Autodesk Inventor part; units mm, degrees
ref_plane "YZ Plane" through (0, 0, 0) normal (1, 0, 0) x (0, 1, 0)
ref_plane "XY Plane" through (0, 0, 0) normal (0, 0, 1) x (1, 0, 0)
sketch "Sketch6" plane through (0, 0, 0) normal (0, 0, 1) x (1, 0, 0)
  arc A0 (-16.2362, 5.1697) -> (-16.2362, -5.1697) centre (-7.62, 0) ccw
  arc A1 (9.9552, 16.756) -> (-16.2362, 5.1697) centre (5.08, -7.62) ccw
  arc A2 (9.9552, -16.756) -> (9.9552, 16.756) centre (6.604, 0) ccw
  line L0 (-27.0242, 0) -> (35.6389, 0)
  arc A3 (-16.2362, 5.1697) -> (-16.2362, -5.1697) centre (-7.62, 0) ccw
  arc A4 (-16.2362, -5.1697) -> (9.9552, -16.756) centre (5.08, 7.62) ccw
  arc A5 (9.9552, -16.756) -> (23.6918, 0) centre (6.604, 0) ccw
  line L1 (0, -29.2695) -> (0, 29.2695)
  circle A6 centre (0, 0) radius 3.175
  dimension "d11" = 7.62
  dimension "d12" = 5.08
  dimension "d13" = 6.35
  dimension "d16" = 6.604
  dimension "d17" = 7.62
extrude "Extrusion2" add sketch "Sketch6" along normal blind 6.35 contours A1 L1 A6 L0 A0 | L0 A6 L1 A4 A0 | A1 A2 L0 A6 L1 | L1 A6 L0 A2 A4
properties part number "Cam disc Polyline"
Input: part model. Units: mm. Frame: model coordinates. Coordinates: 2 decimals unless noted, no trailing zeros. Loops run counter-clockwise (first coordinate to the right, second up) from the corner with the lowest first, then second, coordinate; pieces in that order, holes last. Notation, with made-up numbers: (4.5, 29.5) - (35.5, 29.5) arc R6 cw to (35.5, 38.5) - close; hole circle Ø3 at (-6, -2). An arc over 180 degrees is marked (long way). Answer in a Markdown table with one row per item. Add a question column.
Item 1: Section query B-B on x = 1. Return the cut outline in (y, z).
Item 2: Section query A-A on y = 0. Return the cut outline in (x, z) (3 decimals), then the cut area to 3 significant figures.
Item 3: Section query C-C on z = 3. Return the cut outline in (x, y) (3 decimals).
Item 4: Contact query for flat-ended pins moving along their axis: P1, Ø1, axis at x = 8, z = 3, coming from the +Y side; P2, Ø2, axis at x = 15.5, z = 3.5, coming from the +Y side; P3, Ø1, axis at x = 18.5, z = 3.5, coming from the +Y side. Output: stop coordinate, or through.
Item 5: Section query D-D on y = 12.5. Return the cut outline in (x, z).
Item 6: Line query: line 1 along X through (y, z) = (0, 3.75) (3 decimals); line 2 along Y through (x, z) = (0, 5) (3 decimals); line 3 along X through (y, z) = (-2, 0.5). Output: solid intervals per line, ascending. Write a range as [from, to].
Recorded:
| question | item | result |
|---|---|---|
| 1 | outline | (-16.9, 0) - (-3.01, 0) - (-3.01, 6.35) - (-16.9, 6.35) - close; (3.01, 0) - (16.9, 0) - (16.9, 6.35) - (3.01, 6.35) - close |
| 2 | outline | (-17.668, 0) - (-3.175, 0) - (-3.175, 6.35) - (-17.668, 6.35) - close; (3.175, 0) - (23.692, 0) - (23.692, 6.35) - (3.175, 6.35) - close |
| 2 | area | 222 mm^2 |
| 3 | outline | (-16.236, -5.17) arc R24.859 ccw to (9.955, -16.756) arc R17.088 ccw to (9.955, 16.756) arc R24.859 ccw to (-16.236, 5.17) arc R10.048 ccw to start; hole circle Ø6.35 at (0, 0) |
| 4 | P1 | y = 17.12 |
| 4 | P2 | y = 15.15 |
| 4 | P3 | y = 12.73 |
| 5 | outline | (-9.52, 0) - (18.25, 0) - (18.25, 6.35) - (-9.52, 6.35) - close |
| 6 | line 1 | [-17.668, -3.175], [3.175, 23.692] |
| 6 | line 2 | [-16.714, -3.175], [3.175, 16.714] |
| 6 | line 3 | [-17.47, -2.47], [2.47, 23.57] |
